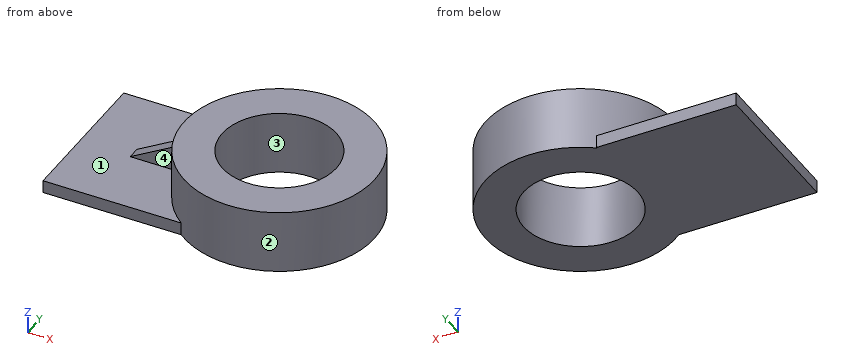
```python
from build123d import *

# Parameters (mm, degrees)
F0_W     = 69.85
F0_H     = 76.2
F1_DEPTH = 6.35
F3_DEPTH = 3.175
F4_R     = 47.625
F4_R_2   = 28.575
F5_DEPTH = 31.75


with BuildPart() as f1:
    # F0 (on Top) → F1 (new body)
    with BuildSketch(Plane.XY):
        with Locations((-34.925, 0.542263)):
            Rectangle(F0_W, F0_H)
    extrude(amount=F1_DEPTH)

    # F2 (on Front) → F3 (join, symmetric)
    with BuildSketch(Plane.XZ):
        Polygon((-44.45, 6.35), (0, 6.35), (0, 31.75), align=None)
    extrude(amount=F3_DEPTH, both=True)

    # F4 (on face) → F5 (join)
    with BuildSketch(Plane(origin=(0, 0, 0), x_dir=(1, 0, 0), z_dir=(0, 0, -1))):
        with Locations((28.575, 0)):
            Circle(F4_R)
        with Locations((28.575, 0)):
            Circle(F4_R_2, mode=Mode.SUBTRACT)
    extrude(amount=-F5_DEPTH)


solid = f1.part
```
Work out the finished part from the listing and answer in its coordinate system (mm). Face numbers are marked on the shaded views. Give positions to 0.01 mm unless a question says otherwise; leave off trailing zeros. Loops run counter-clockwise (first coordinate to the right, second up) from the corner with the lowest first, then second, coordinate; pieces in that order, holes last. Notation, with made-up numbers: (34, -32.75) -> (62, -32.75) arc R20 cw to (62, 5.25) -> close; hole circle Ø8 at (7, 2.5). An arc over 180 degrees is marked (long way). Put each result on its own line as item: value. Start each with the question number.
Item 1: Find the intervals of material crossed by L1, parallel to Z at x = -56, y = -36.5; L2, parallel to Y at x = 21, z = 7; L3, parallel to X at y = -12.5, z = 5, in increasing order. Write a range as [from, to].
Item 2: The part is cut by section C-C (z = 26). Give the vertices of the cut face in (x, y) (3 decimals).
Item 3: The part is cut by section B-B (y = -24.5). Give the vertices of the cut face in (x, z).
Item 4: The mould has two halves that part along Y. Classify the marked faces 1, 2, 3 and 4: released by +Y, released by -Y, zero draft, split by the parting line, or undercut.
Item 5: The part is cut by section D-D (y = 33). Give the vertices of the cut face in (x, z).
Item 6: Each of these flat-tipped pins is pushed along its axis until it touches: P1, Ø1, axis at y = 16.5, z = 18, coming from the -X side; P2, Ø7.5, axis at x = -33, z = 10.5, coming from the +Y side (3 decimals); P3, Ø7, axis at x = -22, z = 1.5, coming from the -Y side. Where does it stop, or does it pass through?
Item 7: The part is cut by section A-A (x = 41). Give the vertices of the cut face in (y, z), then the cut area to 3 significant figures.
Answers below:
1. L1: [0, 6.35]
1. L2: [-47.02, -27.55], [27.55, 47.02]
1. L3: [-69.85, 2.88], [54.27, 74.53]
2. outline: circle Ø95.25 at (28.575, 0); hole circle Ø57.15 at (28.575, 0)
3. outline: (-69.85, 0) -> (13.87, 0) -> (13.87, 31.75) -> (-12.26, 31.75) -> (-12.26, 6.35) -> (-69.85, 6.35) -> close; (43.28, 0) -> (69.41, 0) -> (69.41, 31.75) -> (43.28, 31.75) -> close
4. face 1: zero draft
4. face 2: split by the parting line
4. face 3: undercut
4. face 4: released by -Y
5. outline: (-69.85, 0) -> (62.91, 0) -> (62.91, 31.75) -> (-5.76, 31.75) -> (-5.76, 6.35) -> (-69.85, 6.35) -> close
6. P1: x = -16.28
6. P2: y = 3.175
6. P3: y = -37.56
7. outline: (-45.98, 0) -> (-25.73, 0) -> (-25.73, 31.75) -> (-45.98, 31.75) -> close; (25.73, 0) -> (45.98, 0) -> (45.98, 31.75) -> (25.73, 31.75) -> close
7. area: 1,290 mm2
